The drawing under review shows one solid part. Ordinate dimensions are in mm from its lowest x, y, z. A direction names the side the tool comes from. Round coordinates to 2 decimals unless told otherwise and drop trailing zeros. Order: outer loops, then holes, each group sorted by start corner. A loop starts at its lowest first (then second) coordinate and runs counter-clockwise, first axis right, second up. Notation, with made-up numbers: M 16,2.5 L 29,2.5 A29 ccw 29,31.5 Z; hole C 64,88 d9. An arc over 180 degrees is marked long. Use a Markdown table: item, result.
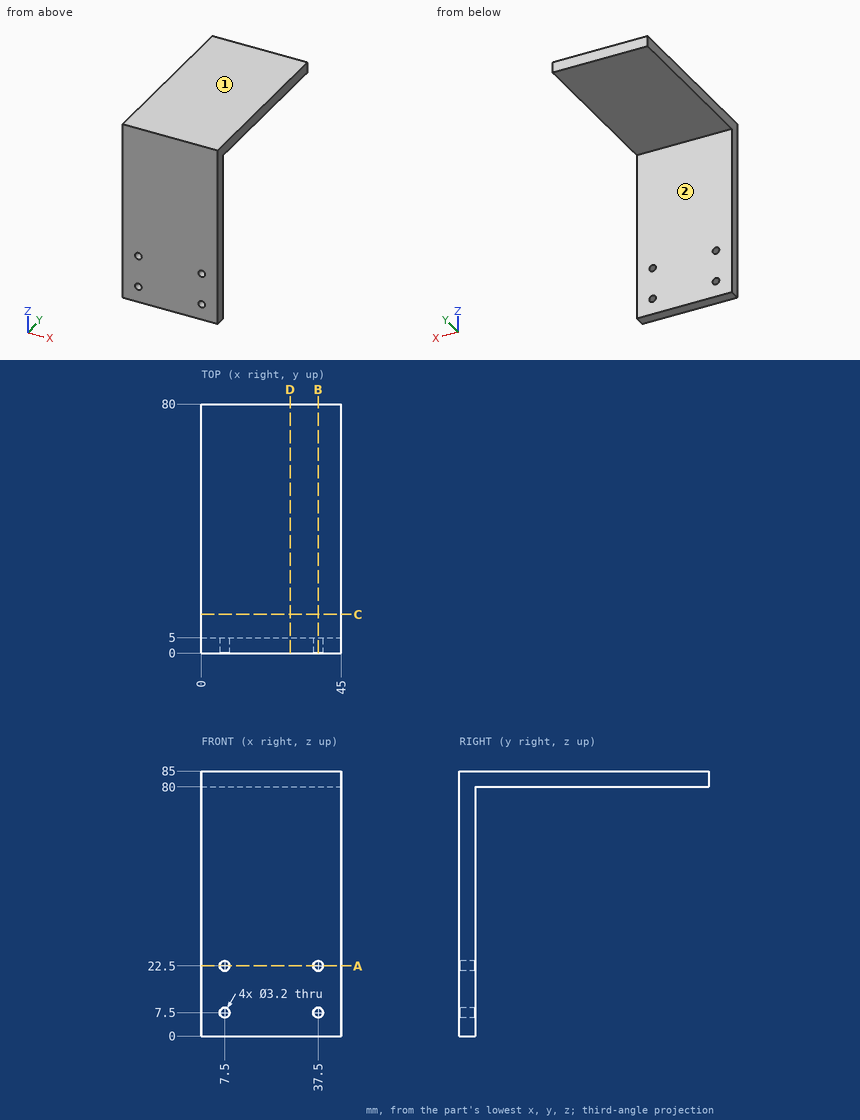
Q1. Add section C-C (y = 12.5). Write out the cut boundary in (x, z).
Determined:
| item | result |
|---|---|
| outline | M 0,80 L 45,80 L 45,85 L 0,85 Z |
Q2. Machinability: for the marked faces 1 and 2, which of the approach directions +Z, -Z, +X, -X, +Y, -Y give a long, thin tool a straight path to every point of the face, cutting with its end or side? Answer none if there is none.
Determined:
| item | result |
|---|---|
| face 1 | +Z, +X, -X, +Y, -Y |
| face 2 | -Z, +X, -X, +Y |
Q3. Add section A-A (z = 22.5). Write out the cut boundary in (x, y).
Determined:
| item | result |
|---|---|
| outline | M 0,0 L 5.9,0 L 5.9,5 L 0,5 Z; M 9.1,0 L 35.9,0 L 35.9,5 L 9.1,5 Z; M 39.1,0 L 45,0 L 45,5 L 39.1,5 Z |
Q4. Add section D-D (x = 28.5). Write out the cut boundary in (y, z), then the cut area to 3 significant figures.
Determined:
| item | result |
|---|---|
| outline | M 0,0 L 5,0 L 5,80 L 80,80 L 80,85 L 0,85 Z |
| area | 800 mm^2 |
Q5. Wall thickness on line 1 along Z through (x, y) = (37.5, 3.6); line 2 along X through (y, z) = (2.1, 22.5); line 3 along Z through (x, y) = (7, 3): over which ranges is each line inside the solid? List them lowest first. Write a range as [from, to].
Determined:
| item | result |
|---|---|
| line 1 | z = [0, 5.9], [9.1, 20.9], [24.1, 85] |
| line 2 | x = [0, 5.9], [9.1, 35.9], [39.1, 45] |
| line 3 | z = [0, 5.98], [9.02, 20.98], [24.02, 85] |
Q6. Clearance check with flat-ended pins moving along their axes: pin 1 (13.5 mm diameter, centred on x = 11.5, z = 42.5, fed in from +Y); pin 2 (22.5 mm diameter, centred on x = 16, y = 48, fed in from -Z). State where each tip first meets the part, or that it passes through.
Determined:
| item | result |
|---|---|
| pin 1 | stops at y = 5 |
| pin 2 | stops at z = 80 |
Q7. Add section B-B (x = 37.5). Write out the cut boundary in (y, z).
Determined:
| item | result |
|---|---|
| outline | M 0,0 L 5,0 L 5,5.9 L 0,5.9 Z; M 0,9.1 L 5,9.1 L 5,20.9 L 0,20.9 Z; M 0,24.1 L 5,24.1 L 5,80 L 80,80 L 80,85 L 0,85 Z |
